```python
from build123d import *

# Parameters (mm, degrees)
F1_W     = 5
F1_H     = 2.5
F1_W_2   = 2.5
F1_H_2   = 5
F2_DEPTH = 15
F5_R     = 5


with BuildPart() as f2:
    # F1 (on Top) → F2 (new body)
    with BuildSketch(Plane.XY):
        with BuildLine():
            ThreePointArc((-26.0240273593, -5), (-26.5, 0), (-26.0240273593, 5))
            Line((-26.0240273593, 5), (-29.5803989155, 5))
            ThreePointArc((-29.5803989155, 5), (-30, 0), (-29.5803989155, -5))
            Line((-29.5803989155, -5), (-26.0240273593, -5))
        make_face()
        with BuildLine():
            Line((-24, 2.5), (-10, 2.5))
            Line((-10, 2.5), (-10, 5))
            Line((-10, 5), (-26.0240273593, 5))
            ThreePointArc((-26.0240273593, 5), (-26.5, 0), (-26.0240273593, -5))
            Line((-26.0240273593, -5), (-10, -5))
            Line((-10, -5), (-10, -2.5))
            Line((-10, -2.5), (-24, -2.5))
            Line((-24, -2.5), (-24, 2.5))
        make_face()
        with BuildLine():
            Line((5, -10), (2.5, -10))
            Line((2.5, -10), (2.5, -24))
            Line((2.5, -24), (-2.5, -24))
            Line((-2.5, -24), (-2.5, -10))
            Line((-2.5, -10), (-5, -10))
            Line((-5, -10), (-5, -26.0240273593))
            ThreePointArc((-5, -26.0240273593), (0, -26.5), (5, -26.0240273593))
            Line((5, -26.0240273593), (5, -10))
        make_face()
        with BuildLine():
            Line((10, 5), (10, 2.5))
            Line((10, 2.5), (24, 2.5))
            Line((24, 2.5), (24, -2.5))
            Line((24, -2.5), (10, -2.5))
            Line((10, -2.5), (10, -5))
            Line((10, -5), (26.0240273593, -5))
            ThreePointArc((26.0240273593, -5), (26.3807384755, -2.5113019509), (26.5, 0))
            ThreePointArc((26.5, 0), (26.3807384755, 2.5113019509), (26.0240273593, 5))
            Line((26.0240273593, 5), (10, 5))
        make_face()
        with BuildLine():
            Line((2.5, 24), (2.5, 10))
            Line((2.5, 10), (5, 10))
            Line((5, 10), (5, 26.0240273593))
            ThreePointArc((5, 26.0240273593), (0, 26.5), (-5, 26.0240273593))
            Line((-5, 26.0240273593), (-5, 10))
            Line((-5, 10), (-2.5, 10))
            Line((-2.5, 10), (-2.5, 24))
            Line((-2.5, 24), (2.5, 24))
        make_face()
        with BuildLine():
            ThreePointArc((-5, 26.0240273593), (0, 26.5), (5, 26.0240273593))
            Line((5, 26.0240273593), (5, 29.5803989155))
            ThreePointArc((5, 29.5803989155), (0, 30), (-5, 29.5803989155))
            Line((-5, 29.5803989155), (-5, 26.0240273593))
        make_face()
        with BuildLine():
            Line((29.5803989155, 5), (26.0240273593, 5))
            ThreePointArc((26.0240273593, 5), (26.3807384755, 2.5113019509), (26.5, 0))
            ThreePointArc((26.5, 0), (26.3807384755, -2.5113019509), (26.0240273593, -5))
            Line((26.0240273593, -5), (29.5803989155, -5))
            ThreePointArc((29.5803989155, -5), (29.8949156836, -2.5087878084), (30, 0))
            ThreePointArc((30, 0), (29.8949156836, 2.5087878084), (29.5803989155, 5))
        make_face()
        with BuildLine():
            ThreePointArc((2.5, 3.4369317712), (3.00520382, 3.00520382), (3.4369317712, 2.5))
            Line((3.4369317712, 2.5), (5, 2.5))
            Line((5, 2.5), (5, 5))
            Line((5, 5), (2.5, 5))
            Line((2.5, 5), (2.5, 3.4369317712))
        make_face()
        with BuildLine():
            ThreePointArc((-2.5, 3.4369317712), (0, 4.25), (2.5, 3.4369317712))
            Line((2.5, 3.4369317712), (2.5, 5))
            Line((2.5, 5), (-2.5, 5))
            Line((-2.5, 5), (-2.5, 3.4369317712))
        make_face()
        with BuildLine():
            ThreePointArc((-3.4369317712, 2.5), (-3.00520382, 3.00520382), (-2.5, 3.4369317712))
            Line((-2.5, 3.4369317712), (-2.5, 5))
            Line((-2.5, 5), (-5, 5))
            Line((-5, 5), (-5, 2.5))
            Line((-5, 2.5), (-3.4369317712, 2.5))
        make_face()
        with BuildLine():
            ThreePointArc((-3.4369317712, -2.5), (-4.25, 0), (-3.4369317712, 2.5))
            Line((-3.4369317712, 2.5), (-5, 2.5))
            Line((-5, 2.5), (-5, -2.5))
            Line((-5, -2.5), (-3.4369317712, -2.5))
        make_face()
        with BuildLine():
            Line((-2.5, -5), (-2.5, -3.4369317712))
            ThreePointArc((-2.5, -3.4369317712), (-3.00520382, -3.00520382), (-3.4369317712, -2.5))
            Line((-3.4369317712, -2.5), (-5, -2.5))
            Line((-5, -2.5), (-5, -5))
            Line((-5, -5), (-2.5, -5))
        make_face()
        with BuildLine():
            Line((2.5, -5), (2.5, -3.4369317712))
            ThreePointArc((2.5, -3.4369317712), (0, -4.25), (-2.5, -3.4369317712))
            Line((-2.5, -3.4369317712), (-2.5, -5))
            Line((-2.5, -5), (2.5, -5))
        make_face()
        with BuildLine():
            Line((5, -2.5), (3.4369317712, -2.5))
            ThreePointArc((3.4369317712, -2.5), (3.00520382, -3.00520382), (2.5, -3.4369317712))
            Line((2.5, -3.4369317712), (2.5, -5))
            Line((2.5, -5), (5, -5))
            Line((5, -5), (5, -2.5))
        make_face()
        with BuildLine():
            ThreePointArc((3.4369317712, 2.5), (4.041624675, 1.3144466464), (4.25, 0))
            ThreePointArc((4.25, 0), (4.041624675, -1.3144466464), (3.4369317712, -2.5))
            Line((3.4369317712, -2.5), (5, -2.5))
            Line((5, -2.5), (5, 2.5))
            Line((5, 2.5), (3.4369317712, 2.5))
        make_face()
        with BuildLine():
            Line((5, -29.5803989155), (5, -26.0240273593))
            ThreePointArc((5, -26.0240273593), (0, -26.5), (-5, -26.0240273593))
            Line((-5, -26.0240273593), (-5, -29.5803989155))
            ThreePointArc((-5, -29.5803989155), (0, -30), (5, -29.5803989155))
        make_face()
        with Locations((-7.5, 3.75)):
            Rectangle(F1_W, F1_H)
        with Locations((7.5, 3.75)):
            Rectangle(F1_W, F1_H)
        with Locations((3.75, -7.5)):
            Rectangle(F1_W_2, F1_H_2)
        with Locations((0, -7.5)):
            Rectangle(F1_W, F1_H_2)
        with Locations((-3.75, -7.5)):
            Rectangle(F1_W_2, F1_H_2)
        with Locations((-7.5, -3.75)):
            Rectangle(F1_W, F1_H)
        with Locations((7.5, -3.75)):
            Rectangle(F1_W, F1_H)
        with Locations((3.75, 7.5)):
            Rectangle(F1_W_2, F1_H_2)
        with Locations((0, 7.5)):
            Rectangle(F1_W, F1_H_2)
        with Locations((-7.5, 0)):
            Rectangle(F1_W, F1_H_2)
        with Locations((7.5, 0)):
            Rectangle(F1_W, F1_H_2)
        with Locations((-3.75, 7.5)):
            Rectangle(F1_W_2, F1_H_2)
    extrude(amount=F2_DEPTH)

    # F3 (on Front) → F4 (revolve, cut)
    with BuildSketch(Plane.XZ):
        Polygon((-30, 15), (-30, 2.7), (-15, 15), align=None)
    revolve(axis=Axis((0, 0, 7.5), (0, 0, 1)), mode=Mode.SUBTRACT)

    # F5
    f5_edges = [f2.edges().sort_by_distance(p)[0] for p in [
        (5, 5, 7.5),
        (5, -5, 7.5),
        (-5, -5, 7.5),
        (-5, 5, 7.5),
    ]]
    fillet(f5_edges, radius=F5_R)


solid = f2.part
```
Geometry check sheet. Reference: the model listing, model coordinates, mm. A direction names the side the tool comes from. Coordinates: 2 decimals unless noted, no trailing zeros. Write each loop counter-clockwise with the first axis right and the second up, starting at its lowest first coordinate (ties: lowest second). Pieces come first, ordered by that corner, then holes. Notation, with made-up numbers: (52.25, 86.25) -> (83.25, 86.25) arc R29 ccw to (83.25, 106.25) -> close; hole circle Ø7 at (-19, 36). An arc over 180 degrees is marked (long way). Use CSV: the item, a comma, the result in double quotes. Start each with the question number.
Item 1: Cross-section at A-A, the plane x = 7. Record the cut outline in (y, z).
Item 2: Depth check by flat-ended pin: pin 1 Ø7.5 at (y, z) = (-17.5, 10) entering from +X; pin 2 Ø2 at (x, y) = (-6.5, -21.5) entering from +Z; pin 3 Ø2.5 at (x, z) = (1, 6) entering from +Y; pin 4 Ø4 at (y, z) = (0, 6) entering from -X. Enter the tip coordinate at first touch or a pass-through.
Item 3: Cross-section at B-B, the plane z = 5.5. State how many separate pieces and enclosed holes the cut face has, plus the area to 3 significant figures.
Item 4: Thickness scan on line 1 (Y direction, x = 14, z = 1.5); line 2 (X direction, y = 1, z = 3.5). Record the ranges inside material, lowest first.
Item 5: Mould release check, pull along X, two halves, no side actions. Record for faces 1 (the flat face through (-17, 5, 6)), 2 (the flat face through (10, 0, 7)), 3 (the cylindrical face through (7, -6, 8)), 4 (the cylindrical face through (-6, 7, 8)): released by +X, released by -X, zero draft, split by the parting line, or undercut.
Item 6: Set-up check for faces 5 (the flat face through (-2.5, -17, 6)), 6 (the flat face through (-18, -5, 6)), 7 (the flat face through (5, 17, 6)), 8 (the flat face through (-5, 18, 6)): record each of +Z, -Z, +X, -X, +Y, -Y from which the full face is reachable in a straight line by a thin tool's end or side.
Answers:
1,outline,"(-6, 0) -> (6, 0) -> (6, 15) -> (-6, 15) -> close"
2,pin 1,"x = 5"
2,pin 2,"through"
2,pin 3,"y = 27.48"
2,pin 4,"x = -28.41"
3,separate pieces,"1"
3,enclosed holes,"5"
3,area,"642 mm^2"
4,line 1,"-5 to -2.5, 2.5 to 5"
4,line 2,"-29.01 to -24, -10 to -4.13, 4.13 to 10, 24 to 29.01"
5,face 1,"zero draft"
5,face 2,"undercut"
5,face 3,"released by +X"
5,face 4,"released by -X"
6,face 5,"+Z, -Z"
6,face 6,"+Z, -Z, -X, -Y"
6,face 7,"+Z, -Z, +X, +Y"
6,face 8,"+Z, -Z, -X, +Y"
